from build123d import *

# Parameters (mm, degrees)
IZIM4_R                     = 55
Y_KSEKLIK_EKSTR_ZYON1_DEPTH = 18.375
KES_EKSTR_ZYON2_DEPTH       = 25
DAIRESEL_KAPLAMA2_COUNT     = 20
KES_EKSTR_ZYON3_DEPTH       = 36.75


with BuildPart() as part:
    # Çizim4 → Yükseklik-Ekstrüzyon1 (new, symmetric)
    with BuildSketch(Plane(origin=(0, 0, 0), x_dir=(1, 0, 0), z_dir=(0, 1, 0))):
        with Locations(Location((0, 0, 0), (0, 0, 270))):
            Circle(IZIM4_R)
    extrude(amount=Y_KSEKLIK_EKSTR_ZYON1_DEPTH, both=True)

    # Çizim2 → Kes-Ekstrüzyon2 (cut, symmetric)
    with BuildSketch(Plane(origin=(0, 0, 0), x_dir=(1, 0, 0), z_dir=(0, 1, 0))):
        with BuildLine():
            ThreePointArc((6.364657179, 54.630496419), (0, 55), (-6.364657179, 54.630496419))
            ThreePointArc((-6.364657179, 54.630496419), (-3.766285823, 49.400564339), (-2.640650949, 43.670235431))
            ThreePointArc((-2.640650949, 43.670235431), (0, 43.75), (2.640650949, 43.670235431))
            ThreePointArc((2.640650949, 43.670235431), (3.766285823, 49.400564339), (6.364657179, 54.630496419))
        make_face()
    kes_ekstr_zyon2 = extrude(amount=KES_EKSTR_ZYON2_DEPTH, both=True, mode=Mode.SUBTRACT)

    # Dairesel Kaplama2: Kes-Ekstrüzyon2 ×20 about axis
    dairesel_kaplama2_axis = Axis((0, 0, 0), (0, 1, 0))
    for i in range(1, DAIRESEL_KAPLAMA2_COUNT):
        add(kes_ekstr_zyon2.rotate(dairesel_kaplama2_axis, i * 360 / DAIRESEL_KAPLAMA2_COUNT), mode=Mode.SUBTRACT)

    # Çizim9 → Kes-Ekstrüzyon3 (cut)
    with BuildSketch(Plane(origin=(0, 18.375, 0), x_dir=(1, 0, 0), z_dir=(0, 1, 0))):
        with BuildLine():
            Line((2.75, 10.58614218), (2.75, 12.833671532))
            ThreePointArc((2.75, 12.833671532), (0, 13.125), (-2.75, 12.833671532))
            Line((-2.75, 12.833671532), (-2.75, 10.58614218))
            ThreePointArc((-2.75, 10.58614218), (0, -10.9375), (2.75, 10.58614218))
        make_face()
    extrude(amount=-KES_EKSTR_ZYON3_DEPTH, mode=Mode.SUBTRACT)


solid = part.part
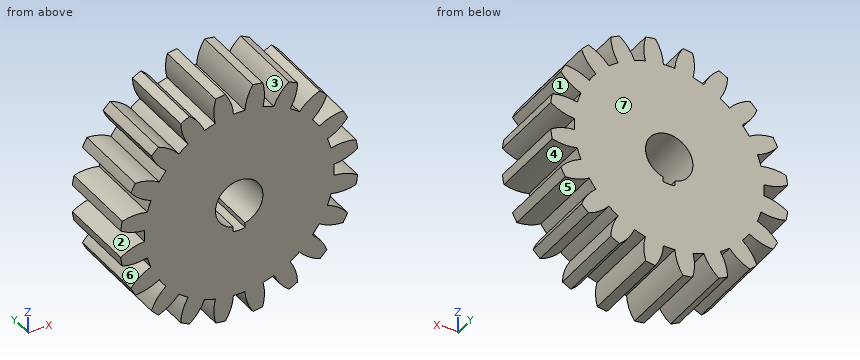
For this review, take the finished solid that the model builds, in its own axes (mm). Face numbers are marked on the shaded views. A direction names the side the tool comes from. Round coordinates to 2 decimals unless told otherwise and drop trailing zeros. Order: outer loops, then holes, each group sorted by start corner. A loop starts at its lowest first (then second) coordinate and runs counter-clockwise, first axis right, second up. Notation, with made-up numbers: M 45.25,55.5 L 90.25,55.5 A12 cw 90.25,59.5 Z; hole C 5.25,-37.5 d7. An arc over 180 degrees is marked long. Write each question's results on one line, items separated by ' | '. Start each with the question number.
1. To check wall thickness, follow L1, parallel to X at y = 8.5, z = 0; L2, parallel to Z at x = 46, y = 5.5; L3, parallel to X at y = 9, z = 34. State the ranges of each line that lie inside material, in increasing order. Write a range as [from, to].
2. Tool access review of the marked faces 1, 2, 3 and 4: name each direction out of +Z, -Z, +X, -X, +Y, -Y from which nothing blocks a thin tool from reaching the whole face with its end or side.
3. Draft analysis for pull direction X (two halves, no side actions). For the marked faces 5, 6 and 7, state which applies: pulls with the +X half, pulls with the -X half, needs draft (parallel to the pull), parting line crosses it, or undercut.
4. Clearance check with flat-ended pins moving along their axes: pin 1 Ø4 at (y, z) = (12.5, 26.5) entering from -X; pin 2 Ø6 at (x, y) = (-23.5, 12.5) entering from -Z; pin 3 Ø12 at (x, y) = (29.5, 8.5) entering from -Z. State where each tip first meets the part, or that it passes through.
5. Add section C-C (x = 17.5). State the section outline as (y, z) points (3 decimals).
Output values:
1) L1: [-43.75, -10.94], [10.94, 43.75] | L2: [-26.81, -18.98], [-11.61, -2.91], [2.91, 11.61], [18.98, 26.81] | L3: [-38.96, -27.99], [-27.53, 27.53], [27.99, 38.96]
2) face 1: +X, +Y, -Y | face 2: -X, +Y, -Y | face 3: +Z, +Y, -Y | face 4: +Y, -Y
3) face 5: undercut | face 6: pulls with the -X half | face 7: needs draft
4) pin 1: x = -49.24 | pin 2: z = -49.99 | pin 3: z = -49.73
5) outline: M -18.375,-43.789 L 18.375,-43.789 L 18.375,43.789 L -18.375,43.789 Z
